Source: CAD feature listing. Evaluate the final solid. Frame: model axes, mm. A direction names the side the tool comes from. Coordinates: 2 decimals unless noted, no trailing zeros. Write each loop counter-clockwise with the first axis right and the second up, starting at its lowest first coordinate (ties: lowest second). Pieces come first, ordered by that corner, then holes. Notation, with made-up numbers: M -36,-26 L -32,-26 A22 cw -32,2 Z; hole C 18.5,25 d3. An arc over 180 degrees is marked long. One line per item, written item: value. Start each with the question number.
Item 1: Cut plane A-A, the plane y = -14. Output: boundary loops of the cut face in (x, z), then the cut area to 3 significant figures.
Item 2: Pin query (flat end, axial travel): P1, Ø1.5, axis at y = -11, z = 2.5, coming from the +X side. Return the tip coordinate at first contact, or that it passes through.
Item 3: Cut plane C-C, the plane z = -3.5. Output: boundary loops of the cut face in (x, y), then the cut area to 3 significant figures.
Item 4: Set-up query: faces 4 (the flat face through (-3.16, -7.6, -1.52)), 5 (the flat face through (17.46, -7, -8)). Return all of +Z, -Z, +X, -X, +Y, -Y with unobstructed straight access to the full face (end or side cutting, diameter ignored); none if empty.
Item 5: Cut plane D-D, the plane x = 8.75. Output: boundary loops of the cut face in (y, z).
Item 6: Ray query, L1, parallel to Z at x = 16.75, y = -7.75; L2, parallel to Z at x = -2.75, y = -9; L3, parallel to Z at x = 7.25, y = -7. Return the intervals inside material, ascending. Write a range as from..to.
Item 7: Mould query, pull axis X, two halves, no side actions, for faces 1 (the cylindrical face through (-2.15, -7.6, -6.26)), 2 (the flat face through (6, -7, -9.824)), 3 (the flat face through (0.883, -7.605, 3.956)). Classes: released by +X, released by -X, zero draft, split by the parting line, or undercut.
Item 8: Cut plane B-B, the plane x = -3. Output: boundary loops of the cut face in (y, z), then the cut area to 3 significant figures.
```python
from build123d import *

# Parameters (mm, degrees)
F0_W     = 22
F0_H     = 17
F1_DEPTH = 15
F2_R     = 2
F3_DEPTH = 33.7
F5_DEPTH = 25
F7_DEPTH = 25


with BuildPart() as f1:
    # F0 (on Front) → F1 (new body)
    with BuildSketch(Plane.XZ):
        with Locations((6.459691, -1.324071)):
            Rectangle(F0_W, F0_H)
    extrude(amount=F1_DEPTH)

    # F2 (on face) → F3 (cut)
    with BuildSketch(Plane.XZ.offset(15)):
        with Locations((16.459691, -4.824071)):
            Circle(F2_R)
        with Locations((-3.540309, -4.824071)):
            Circle(F2_R)
    extrude(amount=-F3_DEPTH, mode=Mode.SUBTRACT)

    # F4 (on face) → F5 (cut)
    with BuildSketch(Plane.XZ.offset(15)):
        Polygon((-4.540309, 0.825076), (6.459691, 7.175929), (-4.540309, 7.175929), align=None)
        Polygon((17.459691, 7.175929), (6.459691, 7.175929), (17.459691, 0.825076), align=None)
    extrude(amount=-F5_DEPTH, mode=Mode.SUBTRACT)

    # F6 (on face) → F7 (cut)
    with BuildSketch(Plane.XZ.offset(15)):
        with BuildLine():
            Line((-1.816008, -3.810768), (-4.540309, 0.825076))
            Line((-4.540309, 0.825076), (-4.540309, -3.092021))
            ThreePointArc((-4.540309, -3.092021), (-3.030111, -2.890242), (-1.816008, -3.810768))
        make_face()
    extrude(amount=-F7_DEPTH, mode=Mode.SUBTRACT)


solid = f1.part
```
From the geometry:
1. outline: M -4.54,-9.82 L 17.46,-9.82 L 17.46,-6.56 A2 cw long 17.46,-3.09 L 17.46,0.83 L 6.46,7.18 L -4.54,0.83 L -1.82,-3.81 A2 cw -4.54,-6.56 Z
1. area: 280 mm²
2. P1: stops at x = 15.86
3. outline: M -2,-15 L 14.96,-15 L 14.96,0 L -2,0 Z
3. area: 254 mm²
4. face 4: -X, +Y, -Y
4. face 5: +Z, -Z, +X, +Y, -Y
5. outline: M -15,-9.82 L 0,-9.82 L 0,5.85 L -15,5.85 Z
6. L1: z = -9.82..-6.8, -2.85..1.23
6. L2: z = -9.82..-6.66, -2.22..1.86
6. L3: z = -9.82..6.72
7. face 1: undercut
7. face 2: zero draft
7. face 3: released by -X
8. outline: M -15,-9.82 L 0,-9.82 L 0,-6.75 L -15,-6.75 Z; M -15,-1.8 L 0,-1.8 L 0,1.71 L -15,1.71 Z
8. area: 98.8 mm²
